Source: CAD feature listing. Evaluate the final solid. Frame: model axes, mm. Face numbers are marked on the shaded views. A direction names the side the tool comes from. Round coordinates to 2 decimals unless told otherwise and drop trailing zeros. Loops run counter-clockwise (first coordinate to the right, second up) from the corner with the lowest first, then second, coordinate; pieces in that order, holes last. Notation, with made-up numbers: M 12,-39 L 71,-39 A5 cw 71,-32 Z; hole C -40,43.5 d2. An arc over 180 degrees is marked long. Answer as CSV lines item,"result". Start each with the question number.
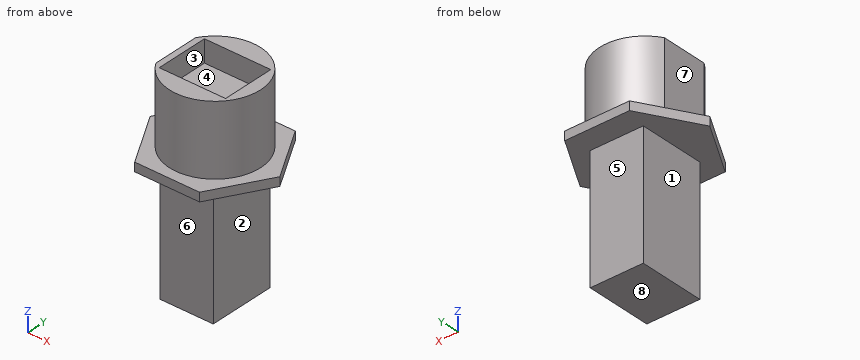
Autodesk Inventor part; units mm, degrees
ref_plane "YZ Plane" through (0, 0, 0) normal (1, 0, 0) x (0, 1, 0)
ref_plane "XZ Plane" through (0, 0, 0) normal (0, 1, 0) x (-1, 0, 0)
ref_plane "XY Plane" through (0, 0, 0) normal (0, 0, 1) x (1, 0, 0)
sketch "Sketch1" plane through (0, 0, 0) normal (0, 0, 1) x (1, 0, 0)
  circle A0 centre (0, 0) radius 10.3188
  line L0 (-8.8812, 5.2536) -> (-8.8812, -5.2536)
  dimension "d0" = 20.6375
  dimension "d10" = 19.2
extrude "Extrusion1" add sketch "Sketch1" along normal blind 16 contours A0 L0 picked at (-2.4812, 0)
sketch "Sketch2" plane through (0, 0, 0) normal (0, 0, -1) x (0, -1, 0)
  line L0 (0, 14.6647) -> (12.7, 7.3323)
  line L1 (12.7, 7.3323) -> (12.7, -7.3323)
  line L2 (12.7, -7.3323) -> (0, -14.6647)
  line L3 (0, -14.6647) -> (-12.7, -7.3323)
  line L4 (-12.7, -7.3323) -> (-12.7, 7.3323)
  line L5 (-12.7, 7.3323) -> (0, 14.6647)
  point P0 (0, 0)
  point P1 (0, 0)
  dimension "d3" = 25.4
extrude "Extrusion2" add sketch "Sketch2" along normal blind 2
sketch "Sketch3" plane through (0, 0, -2) normal (0, 0, -1) x (0, -1, 0)
  line L0 (-7.5, 6) -> (7.5, 6)
  line L1 (7.5, 6) -> (7.5, -6)
  line L2 (7.5, -6) -> (-7.5, -6)
  line L3 (-7.5, -6) -> (-7.5, 6)
  point P0 (0, 0)
  point P1 (-7.5, 0)
  point P2 (0, 6)
  dimension "d6" = 15
  dimension "d7" = 12
extrude "Extrusion3" add sketch "Sketch3" along normal blind 28.2
thread "Thread1"
sketch "Sketch4" plane through (0, 0, 16) normal (0, 0, 1) x (1, 0, 0)
  line L0 (-7.5, 6) -> (7.5, 6)
  line L1 (7.5, 6) -> (7.5, -6)
  line L2 (7.5, -6) -> (-7.5, -6)
  line L3 (-7.5, -6) -> (-7.5, 6)
  point P0 (0, 0)
  point P1 (7.5, 0)
  point P2 (0, 6)
  dimension "d13" = 15
  dimension "d14" = 12
extrude "Extrusion4" cut sketch "Sketch4" against normal blind 5
properties part number "RS PRO Single-Port RJ45 Female Coupler, Shielded"
1) Access query for the marked faces 4, 5, 6, 7 and 8. Directions: +Z, -Z, +X, -X, +Y, -Y. A direction counts if a zero-diameter tool reaches every point of the face in a straight line with its end or side. Return the directions, or none.
2) Ray query, line 1 along Z through (x, y) = (-6, -11); line 2 along X through (y, z) = (-6.5, -15); line 3 along Z through (x, y) = (-3.75, -5). Return the intervals inside material, ascending.
3) Mould query, pull axis X, two halves, no side actions, for the marked faces 1, 2 and 3. Classes: pulls with the +X half, pulls with the -X half, needs draft (parallel to the pull), parting line crosses it, or undercut.
4) Contact query for flat-ended pins moving along their axis: pin 1 Ø4 at (y, z) = (1.5, 13) entering from +X; pin 2 Ø3.5 at (x, z) = (0.5, -16.5) entering from -Y; pin 3 Ø12 at (y, z) = (1, -16) entering from -X. Output: stop coordinate, or through.
5) Section A-A, the plane x = 0. Return loops of the section in (y, z).
6) Section D-D, the plane z = -0.5. Return loops of the section in (x, y).
7) Section B-B, the plane z = 13.5. Return loops of the section in (x, y).
8) Section C-C, the plane y = -8.5. Return loops of the section in (x, z).
Findings below:
1,face 4,"+Z"
1,face 5,"-Z, +X, -X, +Y"
1,face 6,"-Z, +X, -X, -Y"
1,face 7,"+Z, -X, +Y, -Y"
1,face 8,"-Z, +X, -X, +Y, -Y"
2,line 1,"-2 to 0"
2,line 2,"-6 to 6"
2,line 3,"-30.2 to 11"
3,face 1,"pulls with the -X half"
3,face 2,"pulls with the +X half"
3,face 3,"undercut"
4,pin 1,"x = 10.32"
4,pin 2,"y = -7.5"
4,pin 3,"x = -6"
5,outline,"M -12.7,-2 L -7.5,-2 L -7.5,-30.2 L 7.5,-30.2 L 7.5,-2 L 12.7,-2 L 12.7,0 L 10.32,0 L 10.32,16 L 6,16 L 6,11 L -6,11 L -6,16 L -10.32,16 L -10.32,0 L -12.7,0 Z"
6,outline,"M -14.66,0 L -7.33,-12.7 L 7.33,-12.7 L 14.66,0 L 7.33,12.7 L -7.33,12.7 Z"
7,outline,"M -8.88,-5.25 A10.32 ccw long -8.88,5.25 Z; hole M -7.5,-6 L 7.5,-6 L 7.5,6 L -7.5,6 Z"
8,outline,"M -9.76,-2 L 9.76,-2 L 9.76,0 L 5.85,0 L 5.85,16 L -5.85,16 L -5.85,0 L -9.76,0 Z"
